```python
from build123d import *
from OCP.BRepFilletAPI import BRepFilletAPI_MakeChamfer

# Parameters (mm, degrees)
BOSS_EXTRUDE10_DEPTH             = 38
CUT_EXTRUDE7_DEPTH               = 114.357840488
CUT_EXTRUDE7_DEPTH_BACK          = 114.357840488
CUT_EXTRUDE8_REACH               = 164.861
SKETCH44_W                       = 5
SKETCH44_H                       = 3
BOSS_EXTRUDE11_DEPTH             = 13
CHAMFER11_SIZE                   = 3
CHAMFER11_SIZE_2                 = 13
F_2_0_START                      = 25.919230669
F_2_0_2_DIAMETER_HOLE1_OUTLINE_R = 1
F_2_0_2_DIAMETER_HOLE1_DEPTH     = 4.730769331
M4_CLEARANCE_HOLE1_D             = 4.5
F_6_0_6_DIAMETER_HOLE1_D         = 6
FILLET33_R                       = 1
F_3_0_3_DIAMETER_HOLE2_D         = 3
F_3_0_3_DIAMETER_HOLE2_DEPTH     = 2.238381896
SKETCH53_R                       = 75
CUT_EXTRUDE9_DEPTH               = 111.204355799


# Read off the part's stored shape, not the designer's step: Ø2.0 (2) Diameter Hole1
with BuildPart() as part:
    # Sketch34 → Revolve1 (revolve)
    with BuildSketch(Plane.XY, mode=Mode.PRIVATE) as revolve1_sk:
        Polygon((5, 0), (75, 0), (75, 45), (73, 43), (73, 5), (5, 5), align=None)
    revolve(revolve1_sk.sketch.rotate(Axis((0, 0, 0), (0, 1, 0)), 90), axis=Axis((0, 0, 0), (0, 1, 0)))

    # Sketch35 → Boss-Extrude10 (add)
    with BuildSketch(Plane(origin=(0, 5, 0), x_dir=(1, 0, 0), z_dir=(0, 1, 0))):
        with BuildLine():
            Line((-26.551836095, 68), (26.551836095, 68))
            ThreePointArc((26.551836095, 68), (0, 73), (-26.551836095, 68))
        make_face()
        with BuildLine():
            Line((33.226495452, -65), (-33.226495452, -65))
            ThreePointArc((-33.226495452, -65), (0, -73), (33.226495452, -65))
        make_face()
    extrude(amount=BOSS_EXTRUDE10_DEPTH)

    # Sketch36 → Cut-Extrude7 (cut, two sides: drawn at the far end of the back side and taken through both)
    with BuildSketch(Plane(origin=(0, 5, 0), x_dir=(1, 0, 0), z_dir=(0, 1, 0)).offset(-CUT_EXTRUDE7_DEPTH_BACK)):
        with BuildLine():
            Line((-26.551836095, 70.142711667), (26.551836095, 70.142711667))
            ThreePointArc((26.551836095, 70.142711667), (0, 75), (-26.551836095, 70.142711667))
        make_face()
        with BuildLine():
            Line((-33.226495452, -67.238381896), (33.226495452, -67.238381896))
            ThreePointArc((33.226495452, -67.238381896), (0, -75), (-33.226495452, -67.238381896))
        make_face()
    extrude(amount=CUT_EXTRUDE7_DEPTH + CUT_EXTRUDE7_DEPTH_BACK, mode=Mode.SUBTRACT)

    # Sketch43 → Cut-Extrude8 (cut, up to next)
    with BuildSketch(Plane.XY.offset(67.238381896), mode=Mode.PRIVATE) as cut_extrude8_sk1:
        with BuildLine():
            Line((-33.226495452, 29), (33.226495452, 29))
            Line((33.226495452, 29), (33.226495452, 36.795504442))
            ThreePointArc((33.226495452, 36.795504442), (33.791441286, 39.104247508), (35.35861327, 40.891264663))
            Line((35.35861327, 40.891264663), (39.935107214, 44.095760221))
            ThreePointArc((39.935107214, 44.095760221), (41.299460399, 44.768584754), (42.802989396, 45))
            Line((42.802989396, 45), (-42.802989396, 45))
            ThreePointArc((-42.802989396, 45), (-41.299460399, 44.768584754), (-39.935107214, 44.095760221))
            Line((-39.935107214, 44.095760221), (-35.35861327, 40.891264663))
            ThreePointArc((-35.35861327, 40.891264663), (-33.791441286, 39.104247508), (-33.226495452, 36.795504442))
            Line((-33.226495452, 36.795504442), (-33.226495452, 29))
        make_face()
    cut_extrude8_tool1 = extrude(cut_extrude8_sk1.sketch, amount=-CUT_EXTRUDE8_REACH, mode=Mode.PRIVATE) & part.part
    add(cut_extrude8_tool1.solids().sort_by_distance((0, 37.254898, 67.238382))[0], mode=Mode.SUBTRACT)

    # Sketch44 → Boss-Extrude11 (add)
    with BuildSketch(Plane.XY.offset(-68)):
        with Locations((-19.45, 29.15)):
            Rectangle(SKETCH44_W, SKETCH44_H)
        with Locations((8.55, 29.15)):
            Rectangle(SKETCH44_W, SKETCH44_H)
    extrude(amount=BOSS_EXTRUDE11_DEPTH)

    # Chamfer11
    chamfer11_edges_1 = [part.edges().sort_by_distance(p)[0] for p in [
        (8.55, 27.65, -68),
    ]]
    chamfer11_side_1 = [part.faces().sort_by_distance(p)[0] for p in [
        (8.55, 27.59, -68),
    ]]
    chamfer11_edges_2 = [part.edges().sort_by_distance(p)[0] for p in [
        (-19.45, 27.65, -68),
    ]]
    chamfer11_side_2 = [part.faces().sort_by_distance(p)[0] for p in [
        (-19.45, 27.59, -68),
    ]]
    chamfer11 = BRepFilletAPI_MakeChamfer(part.part.solid().wrapped)
    for e in chamfer11_edges_1:
        chamfer11.Add(CHAMFER11_SIZE - 0.0001, CHAMFER11_SIZE_2 - 0.0001, e.wrapped, chamfer11_side_1[0].wrapped)
    for e in chamfer11_edges_2:
        chamfer11.Add(CHAMFER11_SIZE - 0.0001, CHAMFER11_SIZE_2 - 0.0001, e.wrapped, chamfer11_side_2[0].wrapped)
    add(Compound.cast(chamfer11.Shape()), mode=Mode.REPLACE)  # a hair under: the kernel refuses the full size

    # Ø2.0 (2) Diameter Hole1 outline → Ø2.0 (2) Diameter Hole1 (cut)
    with BuildSketch(Plane(origin=(0, 0, 0), x_dir=(1, 0, 0), z_dir=(0, 1, 0)).offset(F_2_0_START)):
        with Locations((8.55, 61.5)):
            Circle(F_2_0_2_DIAMETER_HOLE1_OUTLINE_R)
        with Locations((-19.45, 61.5)):
            Circle(F_2_0_2_DIAMETER_HOLE1_OUTLINE_R)
    extrude(amount=F_2_0_2_DIAMETER_HOLE1_DEPTH, mode=Mode.SUBTRACT)

    # M4 Clearance Hole1 (through all)
    with Locations(Plane(origin=(0, 5, 0), x_dir=(1, 0, 0), z_dir=(0, 1, 0))):
        with Locations((-55, 0), (55, 0), (0, 55), (0, -55)):
            Hole(M4_CLEARANCE_HOLE1_D / 2)

    # Ø6.0 (6) Diameter Hole1 (through all)
    with Locations(Plane(origin=(0, 5, 0), x_dir=(1, 0, 0), z_dir=(0, 1, 0))):
        with Locations((30.0520382, 40.658639918), (40.658639918, 30.0520382), (40.658639918, -30.0520382), (30.0520382, -40.658639918), (-30.0520382, -40.658639918), (-40.658639918, -30.0520382), (-40.658639918, 30.0520382), (-30.0520382, 40.658639918)):
            Hole(F_6_0_6_DIAMETER_HOLE1_D / 2)

    # Fillet33
    fillet33_edges = [part.edges().sort_by_distance(p)[0] for p in [
        (-27.0520382, 5, -40.658639918),
        (-27.0520382, 0, -40.658639918),
        (-37.658639918, 5, -30.0520382),
        (-37.658639918, 0, -30.0520382),
        (-37.658639918, 5, 30.0520382),
        (-37.658639918, 0, 30.0520382),
        (-27.0520382, 5, 40.658639918),
        (-27.0520382, 0, 40.658639918),
        (33.0520382, 5, 40.658639918),
        (33.0520382, 0, 40.658639918),
        (43.658639918, 5, 30.0520382),
        (43.658639918, 0, 30.0520382),
        (43.658639918, 5, -30.0520382),
        (43.658639918, 0, -30.0520382),
        (33.0520382, 5, -40.658639918),
        (33.0520382, 0, -40.658639918),
    ]]
    fillet(fillet33_edges, radius=FILLET33_R)

    # Ø3.0 (3) Diameter Hole2
    with Locations(Plane.XY.offset(67.238381896)):
        with Locations((0, 22), (-15, 8), (15, 8)):
            Hole(F_3_0_3_DIAMETER_HOLE2_D / 2, depth=F_3_0_3_DIAMETER_HOLE2_DEPTH)

    # Sketch53 → Cut-Extrude9 (cut, through all)
    with BuildSketch(Plane(origin=(0, 5, 0), x_dir=(1, 0, 0), z_dir=(0, 1, 0))):
        Circle(SKETCH53_R)
    extrude(amount=-CUT_EXTRUDE9_DEPTH, mode=Mode.SUBTRACT)


solid = part.part
```
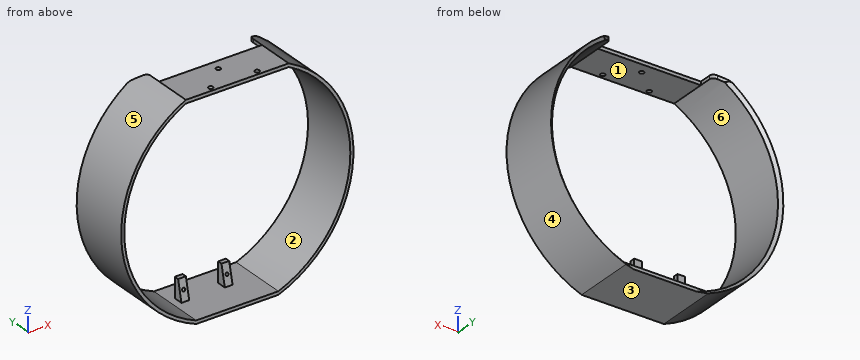
Part model, mm, in its own coordinate system. Face numbers are marked on the shaded views. A direction names the side the tool comes from. Coordinates: 2 decimals unless noted, no trailing zeros. Order: outer loops, then holes, each group sorted by start corner. A loop starts at its lowest first (then second) coordinate and runs counter-clockwise, first axis right, second up. Notation, with made-up numbers: (24.5, 19.5) -> (72.5, 19.5) arc R25 ccw to (72.5, 33.5) -> close; hole circle Ø6 at (29, 35.25). An arc over 180 degrees is marked (long way). Put each result on its own line as item: value. Start each with the question number.
(1) Pin check, flat tips, straight feed: pin 1 Ø2.5 at (x, y) = (-15, 8) entering from +Z; pin 2 Ø3 at (y, z) = (28.5, -62) entering from -X; pin 3 Ø1.5 at (x, y) = (-54, 22.5) entering from +Z; pin 4 Ø12 at (x, z) = (-8.5, -47.5) entering from +Y. Stop position of each tip, or through.
(2) Which spindle directions (+Z, -Z, +X, -X, +Y, -Y) get a long thin tool onto all of the face, cutting with end or side? Do the marked faces 5 and 6. Say none if no direction does.
(3) Probe line 1 along Z through (x, y) = (-11, 23); line 2 along Z through (x, y) = (8.55, 29.4); line 3 along Z through (x, y) = (-19.45, 28.4). List the from-to ranges inside material, lowest first. Write a range as [from, to].
(4) Band-saw the part on A-A (y = 32.5). Give the cut face in (x, z), then the cut area to 3 significant figures.
(5) Mould opens along X. For the marked faces 1, 2, 3 and 4 say: pulls with the +X half, pulls with the -X half, needs draft (parallel to the pull), parting line crosses it, or undercut.
Determined:
1. pin 1: stops at z = -68
1. pin 2: stops at x = -44.33
1. pin 3: stops at z = 52.82
1. pin 4: passes through
2. face 5: -X, +Y, -Y
2. face 6: +Y, -Y
3. line 1: z = [-70.14, -68], [65, 67.24]
3. line 2: z = [-70.14, -62.5], [-60.5, -55]
3. line 3: z = [-70.14, -62.5], [-60.5, -55], [65, 67.24]
4. outline: (-33.23, 65) -> (-33.23, 67.24) arc R75 ccw to (-26.55, -70.14) -> (26.55, -70.14) arc R75 ccw to (33.23, 67.24) -> (33.23, 65) arc R73 cw to (26.55, -68) -> (-26.55, -68) arc R73 cw to start
4. area: 797 mm²
5. face 1: undercut
5. face 2: undercut
5. face 3: needs draft
5. face 4: pulls with the +X half
